Source: CAD feature listing. Evaluate the final solid. Frame: model axes, mm. Face numbers are marked on the shaded views. A direction names the side the tool comes from. Coordinates: 2 decimals unless noted, no trailing zeros. Loops run counter-clockwise (first coordinate to the right, second up) from the corner with the lowest first, then second, coordinate; pieces in that order, holes last.
Item 1: Pull-direction query (X, two-part tool) for the marked faces 1, 2, 3 and 4; classes: +X half, -X half, draft (parallel to the pull), parting line (faces both ways), or undercut.
Item 2: Section query D-D, the plane x = 11.75. Return the cut outline in (y, z), then the cut area to 3 significant figures.
Item 3: Section query B-B, the plane z = -7.5. Return the cut outline in (x, y), then the cut area to 3 significant figures.
Item 4: Line query: probe 1 along Y at (x, z) = (11.5, -6); probe 2 along Z at (x, y) = (7.25, 6). Output: solid intervals per line, ascending.
Item 5: Pin query (flat end, axial travel): pin 1 Ø1.5 at (x, y) = (9, 3.5) entering from -Z; pin 2 Ø5 at (x, z) = (9.5, -3) entering from -Y; pin 3 Ø6.5 at (x, z) = (10.06, 0) entering from -Y. Return the tip coordinate at first contact, or that it passes through.
Item 6: Section query A-A, the plane z = 0. Return the cut outline in (x, y).
Item 7: Reachability of the marked faces 5, 6 and 7 from +Z, -Z, +X, -X, +Y, -Y: full face, straight path, thin tool, end or side. Return the list, or none.
Item 8: Section query C-C, the plane y = 3. Return the cut outline in (x, z).
```python
from build123d import *

# Parameters (mm, degrees)
PAD_DEPTH        = 12.5
HOLE_D           = 2.5
HOLE_DEPTH       = 25
HOLE_CBORE_D     = 5
HOLE_CBORE_DEPTH = 3
SKETCH002_R      = 3.25
HOLE001_DEPTH    = 3.4
CHAMFER_SIZE     = 1


with BuildPart() as part:
    # Sketch → Pad (new body, symmetric)
    with BuildSketch(Plane.XY):
        Polygon((16.124356, 0), (13.093267, 5.25), (7.031089, 5.25), (4, 0), (0, 0), (0, 10.05), (20.124356, 10.05), (20.124356, 0), align=None)
    extrude(amount=PAD_DEPTH, both=True)

    # Hole
    with Locations(Plane.XZ.offset(-5.25)):
        with Locations((10.062178, 0)):
            CounterBoreHole(HOLE_D / 2, HOLE_CBORE_D / 2, HOLE_CBORE_DEPTH, depth=HOLE_DEPTH)

    # Sketch002 (on Face3 of Hole) → Hole001 (cut)
    with BuildSketch(Plane.XZ.offset(-5.65)):
        with Locations((10.062178, 7.5)):
            Circle(SKETCH002_R)
        with Locations((10.062178, -7.5)):
            Circle(SKETCH002_R)
    extrude(amount=-HOLE001_DEPTH, mode=Mode.SUBTRACT)

    # Chamfer
    chamfer_edges = [part.edges().sort_by_distance(p)[0] for p in [
        (2, 0, 12.5),
        (5.515544, 2.625, 12.5),
        (10.062178, 5.25, 12.5),
        (14.608811, 2.625, 12.5),
        (18.124356, 0, 12.5),
        (20.124356, 5.025, 12.5),
        (0, 5.025, 12.5),
        (4, 0, 0),
        (0, 0, 0),
        (20.124356, 0, 0),
        (16.124356, 0, 0),
        (18.124356, 0, -12.5),
        (20.124356, 5.025, -12.5),
        (14.608811, 2.625, -12.5),
        (10.062178, 5.25, -12.5),
        (5.515544, 2.625, -12.5),
        (2, 0, -12.5),
        (0, 5.025, -12.5),
    ]]
    chamfer(chamfer_edges, length=CHAMFER_SIZE)


solid = part.part
```
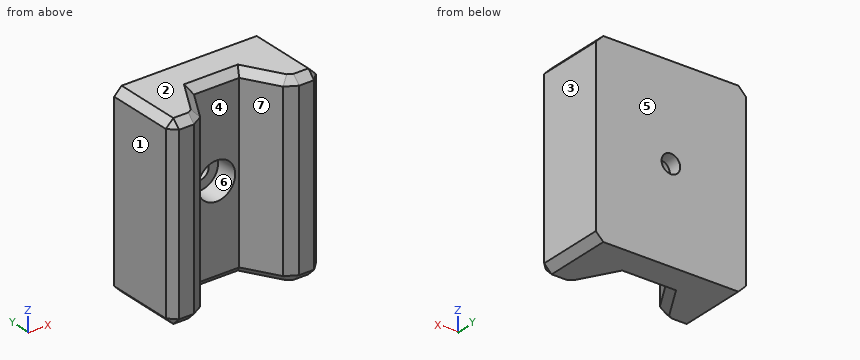
Verdict:
1. face 1: -X half
1. face 2: draft
1. face 3: +X half
1. face 4: undercut
2. outline: (5.25, -11.5) - (6.25, -12.5) - (10.05, -12.5) - (10.05, 12.5) - (6.25, 12.5) - (5.25, 11.5) - (5.25, 1.84) - (8.25, 1.84) - (8.25, -1.84) - (5.25, -1.84) - close; hole (5.65, -10.28) - (9.05, -10.28) - (9.05, -4.72) - (5.65, -4.72) - close; hole (5.65, 4.72) - (9.05, 4.72) - (9.05, 10.28) - (5.65, 10.28) - close
2. area: 70.2 mm2
3. outline: (0, 1) - (1, 0) - (3, 0) - (4.5, 0.87) - (7.03, 5.25) - (13.09, 5.25) - (15.62, 0.87) - (17.12, 0) - (19.12, 0) - (20.12, 1) - (20.12, 10.05) - (0, 10.05) - close; hole (6.81, 5.65) - (13.31, 5.65) - (13.31, 9.05) - (6.81, 9.05) - close
3. area: 131 mm2
4. probe 1: y = 5.25 to 5.65, 9.05 to 10.05
4. probe 2: z = -12.25 to -9.13, -5.87 to 5.87, 9.13 to 12.25
5. pin 1: passes through
5. pin 2: stops at y = 5.2
5. pin 3: stops at y = 4.87
6. outline: (0, 1) - (1, 0) - (3, 0) - (4.5, 0.87) - (7.03, 5.25) - (7.56, 5.25) - (7.56, 8.25) - (8.81, 8.25) - (8.81, 10.05) - (0, 10.05) - close; (11.31, 8.25) - (12.56, 8.25) - (12.56, 5.25) - (13.09, 5.25) - (15.62, 0.87) - (17.12, 0) - (19.12, 0) - (20.12, 1) - (20.12, 10.05) - (11.31, 10.05) - close
7. face 5: +Z, -Z, +X, -X, +Y
7. face 6: -Y
7. face 7: +Z, -Z, -Y
8. outline: (0, -11.5) - (1, -12.5) - (4.58, -12.5) - (5.73, -11.5) - (5.73, 11.5) - (4.58, 12.5) - (1, 12.5) - (0, 11.5) - close; (14.39, -11.5) - (15.55, -12.5) - (19.12, -12.5) - (20.12, -11.5) - (20.12, 11.5) - (19.12, 12.5) - (15.55, 12.5) - (14.39, 11.5) - close
